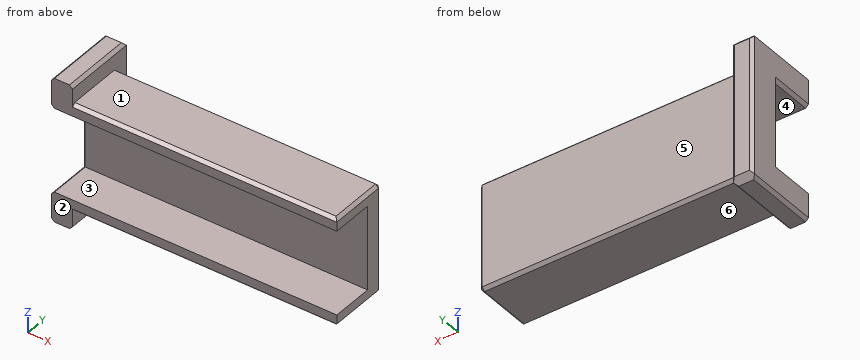
```python
from build123d import *

# Parameters (mm, degrees)
SKETCH_1_W          = 47.45
SKETCH_1_H          = 18
EXTRUDE_1_DEPTH     = 10
SKETCH_2_W          = 24
SKETCH_2_H          = 12.8
EXTRUDE_2_DEPTH     = 3.5
SKETCH_3_W          = 14
SKETCH_3_H          = 7
CUT_EXTRUDE_1_DEPTH = 47.45
CHAMFER_1_SIZE      = 1
CHAMFER_2_SIZE      = 0.5


with BuildPart() as part:
    # 草图1 → 凸台-拉伸1 (new body)
    with BuildSketch(Plane(origin=(0, 0, 0), x_dir=(1, 0, 0), z_dir=(0, 1, 0))):
        Rectangle(SKETCH_1_W, SKETCH_1_H)
    extrude(amount=EXTRUDE_1_DEPTH)

    # 草图2 → 凸台-拉伸2 (add)
    with BuildSketch(Plane.ZY.offset(23.725)):
        with Locations((0, 6.4)):
            Rectangle(SKETCH_2_W, SKETCH_2_H)
    extrude(amount=-EXTRUDE_2_DEPTH)

    # 草图3 → 切除-拉伸1 (cut)
    with BuildSketch(Plane.ZY.offset(23.725)):
        with Locations((0, 3.5)):
            Rectangle(SKETCH_3_W, SKETCH_3_H)
    extrude(amount=-CUT_EXTRUDE_1_DEPTH, mode=Mode.SUBTRACT)

    # 倒角1
    chamfer_1_edges = [part.edges().sort_by_distance(p)[0] for p in [
        (-21.975, 12.8, -12),
        (-21.975, 12.8, 12),
    ]]
    chamfer(chamfer_1_edges, length=CHAMFER_1_SIZE)

    # 倒角2
    chamfer_2_edges = [part.edges().sort_by_distance(p)[0] for p in [
        (1.75, 0, 9),
        (1.75, 0, -9),
        (1.75, 10, -9),
        (1.75, 10, 9),
        (23.725, 5, -9),
        (23.725, 10, 0),
        (23.725, 5, 9),
        (-20.225, 5.9, -12),
        (-20.225, 12.8, 0),
        (-20.225, 5.9, 12),
        (-23.725, 12.8, 0),
        (-23.725, 5.9, -12),
        (-23.725, 5.9, 12),
        (-23.725, 3.5, 7),
        (-23.725, 7, 0),
        (-23.725, 3.5, -7),
    ]]
    chamfer(chamfer_2_edges, length=CHAMFER_2_SIZE - 0.0001)  # a hair under: the kernel refuses the full size


solid = part.part
```
Read the model definition and answer for the solid it produces. Units are mm, in the model's axes. Face numbers are marked on the shaded views. A direction names the side the tool comes from. Round coordinates to 2 decimals unless told otherwise and drop trailing zeros. Write each loop counter-clockwise with the first axis right and the second up, starting at its lowest first coordinate (ties: lowest second). Pieces come first, ordered by that corner, then holes. Notation, with made-up numbers: (-40, 18.5) -> (-30, 18.5) arc R26 ccw to (-30, 56.5) -> close; hole circle Ø5 at (40.5, 59). An arc over 180 degrees is marked (long way). Answer in a Markdown table with one row per item. Add a question column.
1) Find section A-A, the plane y = 3.5. Determine the outline of the cut face in (x, z) (3 decimals), and give its area (3 significant figures).
2) Find section C-C, the plane z = -1.75. Determine the outline of the cut face in (x, y) (3 decimals), and give its area (3 significant figures).
3) Which of the six approach directions +Z, -Z, +X, -X, +Y, -Y give full straight-line access (tool end or side, diameter ignored) to the marked faces 4, 5 and 6?
4) Find section B-B, the plane x = -4.5. Determine the outline of the cut face in (y, z).
5) Consider line 1 (Z direction, x = -15, y = 5.5); line 2 (Y direction, x = -15, z = -4.25); line 3 (Y direction, x = -7, z = 8.5). Determine where each line is inside the solid, lowest interval first.
6) Find section D-D, the plane z = 9.75. Determine the outline of the cut face in (x, y) (3 decimals), and give its area (4 significant figures).
7) Given P1, Ø5, axis at x = 12, y = 3.5, coming from the -Z side; P2, Ø4, axis at x = 9, z = 3, coming from the +Y side; P3, Ø4, axis at x = 0, z = -3.5, coming from the -Y side, each flat-ended and moving along its own axis, determine where each tip first touches the part or whether it passes through.
8) Determine the mould class of the marked faces 1, 2 and 3 for opening direction Z: pulls with the +Z half, pulls with the -Z half, needs draft (parallel to the pull), parting line crosses it, or undercut.
Findings below:
| question | item | result |
|---|---|---|
| 1 | outline | (-23.725, -11.5) -> (-23.225, -12) -> (-20.725, -12) -> (-20.225, -11.5) -> (-20.225, -9) -> (23.225, -9) -> (23.725, -8.5) -> (23.725, -7) -> (-23.225, -7) -> (-23.725, -7.5) -> close; (-23.725, 7.5) -> (-23.225, 7) -> (23.725, 7) -> (23.725, 8.5) -> (23.225, 9) -> (-20.225, 9) -> (-20.225, 11.5) -> (-20.725, 12) -> (-23.225, 12) -> (-23.725, 11.5) -> close |
| 1 | area | 210 mm² |
| 2 | outline | (-23.725, 7.5) -> (-23.225, 7) -> (23.725, 7) -> (23.725, 9.5) -> (23.225, 10) -> (-20.225, 10) -> (-20.225, 12.3) -> (-20.725, 12.8) -> (-23.225, 12.8) -> (-23.725, 12.3) -> close |
| 2 | area | 152 mm² |
| 3 | face 4 | +X, -X, -Y |
| 3 | face 5 | +Z, -Z, +X, +Y |
| 3 | face 6 | -Z, +X, +Y, -Y |
| 4 | outline | (0, -8.5) -> (0.5, -9) -> (9.5, -9) -> (10, -8.5) -> (10, 8.5) -> (9.5, 9) -> (0.5, 9) -> (0, 8.5) -> (0, 7) -> (7, 7) -> (7, -7) -> (0, -7) -> close |
| 5 | line 1 | -9 to -7, 7 to 9 |
| 5 | line 2 | 7 to 10 |
| 5 | line 3 | 0 to 10 |
| 6 | outline | (-23.725, 0) -> (-20.225, 0) -> (-20.225, 12.3) -> (-20.725, 12.8) -> (-23.225, 12.8) -> (-23.725, 12.3) -> close |
| 6 | area | 44.55 mm² |
| 7 | P1 | z = -9 |
| 7 | P2 | y = 10 |
| 7 | P3 | y = 7 |
| 8 | face 1 | pulls with the +Z half |
| 8 | face 2 | needs draft |
| 8 | face 3 | undercut |
